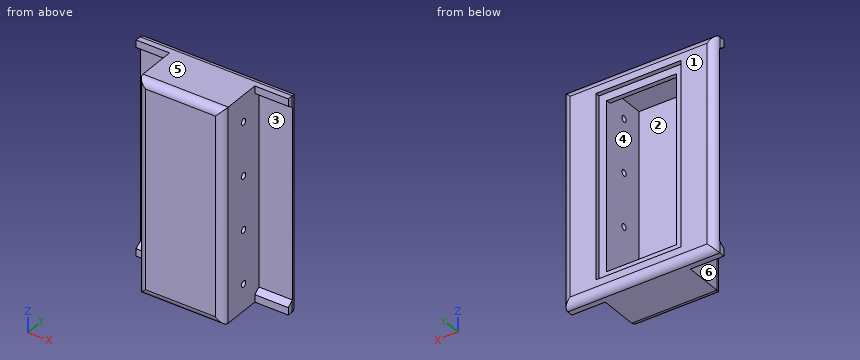
```python
from build123d import *

# Parameters (mm, degrees)
SKETCH1_W           = 200
SKETCH1_H           = 150
BOSS_EXTRUDE1_DEPTH = 280
SKETCH2_W           = 44
SKETCH2_H           = 60
SKETCH2_W_2         = 34
SKETCH2_H_2         = 72.5
CUT_EXTRUDE1_DEPTH  = 280
CUT_EXTRUDE5_DEPTH  = 200
CUT_EXTRUDE8_DEPTH  = 44
CUT_EXTRUDE9_DEPTH  = 44
SKETCH6_W           = 112
SKETCH6_H           = 52.5
CUT_EXTRUDE7_DEPTH  = 280
FILLET1_START       = -100
FILLET1_DEPTH       = 200
FILLET1_START_2     = -76
FILLET1_2_DEPTH     = 10
FILLET1_START_3     = 66
FILLET1_3_DEPTH     = 10
FILLET1_START_4     = -66
FILLET1_4_DEPTH     = 132
FILLET1_START_5     = -281
FILLET1_5_DEPTH     = 282
SKETCH8_W           = 152
SKETCH8_H           = 72.5
CUT_EXTRUDE10_DEPTH = 280
SKETCH9_W           = 111.98598877
SKETCH9_H           = 241.482238642
SKETCH9_W_2         = 91.98598877
SKETCH9_H_2         = 221.482238642
SKETCH9_H_3         = 10
CUT_EXTRUDE11_DEPTH = 6
SKETCH9_3_W         = 45.992994385
SKETCH9_3_H         = 221.482238642
CUT_EXTRUDE12_DEPTH = 67
CUT_EXTRUDE13_START = -12
SKETCH9_7_W         = 91.98598877
SKETCH9_7_H         = 9.258880679
CUT_EXTRUDE13_DEPTH = 55
CUT_EXTRUDE14_START = -12
SKETCH9_9_W         = 91.98598877
SKETCH9_9_H         = 10
CUT_EXTRUDE14_DEPTH = 55
CUT_EXTRUDE15_REACH = 331.182
SKETCH11_R          = 4


with BuildPart() as part:
    # Sketch1 → Boss-Extrude1 (new body)
    with BuildSketch(Plane.XY):
        Rectangle(SKETCH1_W, SKETCH1_H)
    extrude(amount=-BOSS_EXTRUDE1_DEPTH)

    # Sketch2 → Cut-Extrude1 (cut)
    with BuildSketch(Plane.XY):
        with Locations((78, -45)):
            Rectangle(SKETCH2_W, SKETCH2_H)
        with Locations((-78, -45)):
            Rectangle(SKETCH2_W, SKETCH2_H)
        with Locations((83, 38.75)):
            Rectangle(SKETCH2_W_2, SKETCH2_H_2)
        with Locations((-83, 38.75)):
            Rectangle(SKETCH2_W_2, SKETCH2_H_2)
    extrude(amount=-CUT_EXTRUDE1_DEPTH, mode=Mode.SUBTRACT)

    # Sketch3 → Cut-Extrude5 (cut)
    with BuildSketch(Plane.ZY.offset(100)):
        Polygon((-280, 2.5), (-274.399041425, 2.5), (-252, 2.5), (-218.971094498, 75), (-280, 75), align=None)
        Polygon((-236.455453487, 12.5), (-168.766953205, 12.5), (-60.438488841, 12.5), (-94.602997447, 65), (-144.84946991, 65), (-212.537970192, 65), align=None)
        Polygon((-89.179559504, 75), (-42, 2.5), (-5.600958575, 2.5), (0, 2.5), (0, 75), align=None)
    extrude(amount=-CUT_EXTRUDE5_DEPTH, mode=Mode.SUBTRACT)

    # Sketch5 → Cut-Extrude8 (cut)
    with BuildSketch(Plane.ZY.offset(100)):
        Polygon((-264.773291637, -7.125749789), (-270.374250211, -15), (-140, -15), (-140, -7.125749789), align=None)
        Polygon((-15.226708363, -7.125749789), (-140, -7.125749789), (-140, -15), (-9.625749789, -15), align=None)
    extrude(amount=-CUT_EXTRUDE8_DEPTH, mode=Mode.SUBTRACT)

    # Sketch7 → Cut-Extrude9 (cut)
    with BuildSketch(Plane(origin=(100, 0, 0), x_dir=(0, 0, -1), z_dir=(1, 0, 0))):
        Polygon((9.625749789, -15), (15.226708363, -7.125749789), (264.773291637, -7.125749789), (270.374250211, -15), align=None)
    extrude(amount=-CUT_EXTRUDE9_DEPTH, mode=Mode.SUBTRACT)

    # Sketch6 → Cut-Extrude7 (cut)
    with BuildSketch(Plane.XY):
        with Locations((0, 38.75)):
            Rectangle(SKETCH6_W, SKETCH6_H)
    extrude(amount=-CUT_EXTRUDE7_DEPTH, mode=Mode.SUBTRACT)

    # Fillet1: read off the stored shape, not the designer's step
    # Fillet1 outline → Fillet1 (cut)
    with BuildSketch(Plane.YZ.offset(FILLET1_START)):
        with BuildLine():
            Line((-75, 0), (-75, -10))
            ThreePointArc((-75, -10), (-72.071067812, -2.928932188), (-65, 0))
            Line((-65, 0), (-75, 0))
        make_face()
        with BuildLine():
            ThreePointArc((-65, -280), (-72.071067812, -277.071067812), (-75, -270))
            Line((-75, -270), (-75, -280))
            Line((-75, -280), (-65, -280))
        make_face()
        with BuildLine():
            Line((2.5, 0), (-7.5, 0))
            ThreePointArc((-7.5, 0), (-0.428932188, -2.928932188), (2.5, -10))
            Line((2.5, -10), (2.5, 0))
        make_face()
        with BuildLine():
            ThreePointArc((2.5, -270), (-0.428932188, -277.071067812), (-7.5, -280))
            Line((-7.5, -280), (2.5, -280))
            Line((2.5, -280), (2.5, -270))
        make_face()
        with BuildLine():
            Line((75, -89.179559504), (70.454316835, -86.221444616))
            ThreePointArc((70.454316835, -86.221444616), (73.790425711, -89.835564613), (75, -94.602997447))
            Line((75, -94.602997447), (75, -89.179559504))
        make_face()
        with BuildLine():
            ThreePointArc((75, -212.537970192), (73.410042611, -217.948255145), (69.145763344, -221.638115591))
            Line((69.145763344, -221.638115591), (75, -218.971094498))
            Line((75, -218.971094498), (75, -212.537970192))
        make_face()
    extrude(amount=FILLET1_DEPTH, mode=Mode.SUBTRACT)

    # Fillet1 2 outline → Fillet1 2 (add)
    with BuildSketch(Plane.YZ.offset(FILLET1_START_2)):
        with BuildLine():
            ThreePointArc((7.045683165, -44.958114888), (3.709574289, -41.343994891), (2.5, -36.576562057))
            Line((2.5, -36.576562057), (2.5, -258.433124306))
            ThreePointArc((2.5, -258.433124306), (4.089957389, -253.022839352), (8.354236656, -249.332978906))
            Line((8.354236656, -249.332978906), (69.145763344, -221.638115591))
            ThreePointArc((69.145763344, -221.638115591), (73.410042611, -217.948255145), (75, -212.537970192))
            Line((75, -212.537970192), (75, -94.602997447))
            ThreePointArc((75, -94.602997447), (73.790425711, -89.835564613), (70.454316835, -86.221444616))
            Line((70.454316835, -86.221444616), (7.045683165, -44.958114888))
        make_face()
    extrude(amount=FILLET1_2_DEPTH)

    # Fillet1 3 outline → Fillet1 3 (add)
    with BuildSketch(Plane.YZ.offset(FILLET1_START_3)):
        with BuildLine():
            ThreePointArc((7.045683165, -44.958114888), (3.709574289, -41.343994891), (2.5, -36.576562057))
            Line((2.5, -36.576562057), (2.5, -258.433124306))
            ThreePointArc((2.5, -258.433124306), (4.089957389, -253.022839352), (8.354236656, -249.332978906))
            Line((8.354236656, -249.332978906), (69.145763344, -221.638115591))
            ThreePointArc((69.145763344, -221.638115591), (73.410042611, -217.948255145), (75, -212.537970192))
            Line((75, -212.537970192), (75, -94.602997447))
            ThreePointArc((75, -94.602997447), (73.790425711, -89.835564613), (70.454316835, -86.221444616))
            Line((70.454316835, -86.221444616), (7.045683165, -44.958114888))
        make_face()
    extrude(amount=FILLET1_3_DEPTH)

    # Fillet1 4 outline → Fillet1 4 (add)
    with BuildSketch(Plane.YZ.offset(FILLET1_START_4)):
        with BuildLine():
            ThreePointArc((7.045683165, -44.958114888), (3.709574289, -41.343994891), (2.5, -36.576562057))
            Line((2.5, -36.576562057), (2.5, -42))
            Line((2.5, -42), (7.045683165, -44.958114888))
        make_face()
        with BuildLine():
            Line((2.5, -252), (2.5, -258.433124306))
            ThreePointArc((2.5, -258.433124306), (4.089957389, -253.022839352), (8.354236656, -249.332978906))
            Line((8.354236656, -249.332978906), (2.5, -252))
        make_face()
    extrude(amount=FILLET1_4_DEPTH)

    # Fillet1 5 outline → Fillet1 5 (cut)
    with BuildSketch(Plane.XY.offset(FILLET1_START_5)):
        with BuildLine():
            ThreePointArc((56, 75), (63.071067812, 72.071067812), (66, 65))
            Line((66, 65), (66, 12.5))
            ThreePointArc((66, 12.5), (68.928932188, 5.428932188), (76, 2.5))
            Line((76, 2.5), (76, 75))
            Line((76, 75), (56, 75))
        make_face()
        with BuildLine():
            ThreePointArc((-66, 65), (-63.071067812, 72.071067812), (-56, 75))
            Line((-56, 75), (-76, 75))
            Line((-76, 75), (-76, 2.5))
            ThreePointArc((-76, 2.5), (-68.928932188, 5.428932188), (-66, 12.5))
            Line((-66, 12.5), (-66, 65))
        make_face()
        with BuildLine():
            Line((100, 2.5), (90, 2.5))
            ThreePointArc((90, 2.5), (97.071067812, -0.428932188), (100, -7.5))
            Line((100, -7.5), (100, 2.5))
        make_face()
        with BuildLine():
            Line((-90, 2.5), (-100, 2.5))
            Line((-100, 2.5), (-100, -7.5))
            ThreePointArc((-100, -7.5), (-97.071067812, -0.428932188), (-90, 2.5))
        make_face()
        with BuildLine():
            Line((56, -75), (56, -65))
            ThreePointArc((56, -65), (53.071067812, -72.071067812), (46, -75))
            Line((46, -75), (56, -75))
        make_face()
        with BuildLine():
            ThreePointArc((-46, -75), (-53.071067812, -72.071067812), (-56, -65))
            Line((-56, -65), (-56, -75))
            Line((-56, -75), (-46, -75))
        make_face()
    extrude(amount=FILLET1_5_DEPTH, mode=Mode.SUBTRACT)

    # Sketch8 → Cut-Extrude10 (cut)
    with BuildSketch(Plane.XY):
        with Locations((0, 38.75)):
            Rectangle(SKETCH8_W, SKETCH8_H)
    extrude(amount=-CUT_EXTRUDE10_DEPTH, mode=Mode.SUBTRACT)

    # Sketch9 → Cut-Extrude11 (cut)
    # profile 1 of 4: a face of its own
    with BuildSketch(Plane(origin=(0, 2.5, 0), x_dir=(1, 0, 0), z_dir=(0, 1, 0))):
        with Locations((0, 140)):
            Rectangle(SKETCH9_W, SKETCH9_H)
        with Locations((0, 140)):
            Rectangle(SKETCH9_W_2, SKETCH9_H_2, mode=Mode.SUBTRACT)
    # profile 2 of 4: a face of its own
    with BuildSketch(Plane(origin=(0, 2.5, 0), x_dir=(1, 0, 0), z_dir=(0, 1, 0))):
        Polygon((55.992994385, 260.741119321), (45.992994385, 260.741119321), (45.992994385, 250.741119321), (45.992994385, 29.258880679), (45.992994385, 19.258880679), (55.992994385, 19.258880679), align=None)
    # profile 3 of 4: a face of its own
    with BuildSketch(Plane(origin=(0, 2.5, 0), x_dir=(1, 0, 0), z_dir=(0, 1, 0))):
        with Locations((0, 255.741119321)):
            Rectangle(SKETCH9_W_2, SKETCH9_H_3)
    # profile 4 of 4: a face of its own
    with BuildSketch(Plane(origin=(0, 2.5, 0), x_dir=(1, 0, 0), z_dir=(0, 1, 0))):
        with Locations((0, 24.258880679)):
            Rectangle(SKETCH9_W_2, SKETCH9_H_3)
    extrude(amount=-CUT_EXTRUDE11_DEPTH, mode=Mode.SUBTRACT)

    # Sketch9<3> → Cut-Extrude12 (cut)
    with BuildSketch(Plane(origin=(0, 2.5, 0), x_dir=(1, 0, 0), z_dir=(0, 1, 0))):
        with Locations((-22.996497193, 140)):
            Rectangle(SKETCH9_3_W, SKETCH9_3_H)
        with Locations((22.996497193, 140)):
            Rectangle(SKETCH9_3_W, SKETCH9_3_H)
    extrude(amount=-CUT_EXTRUDE12_DEPTH, mode=Mode.SUBTRACT)

    # Sketch9<7> → Cut-Extrude13 (cut)
    with BuildSketch(Plane(origin=(0, 2.5, 0), x_dir=(1, 0, 0), z_dir=(0, 1, 0)).offset(CUT_EXTRUDE13_START)):
        with Locations((0, 265.370559661)):
            Rectangle(SKETCH9_7_W, SKETCH9_7_H)
        with Locations((0, 14.62944034)):
            Rectangle(SKETCH9_7_W, SKETCH9_7_H)
    extrude(amount=-CUT_EXTRUDE13_DEPTH, mode=Mode.SUBTRACT)

    # Sketch9<9> → Cut-Extrude14 (cut)
    with BuildSketch(Plane(origin=(0, 2.5, 0), x_dir=(1, 0, 0), z_dir=(0, 1, 0)).offset(CUT_EXTRUDE14_START)):
        with Locations((0, 255.741119321)):
            Rectangle(SKETCH9_9_W, SKETCH9_9_H)
        with Locations((0, 24.258880679)):
            Rectangle(SKETCH9_9_W, SKETCH9_9_H)
    extrude(amount=-CUT_EXTRUDE14_DEPTH, mode=Mode.SUBTRACT)

    # Cut-Extrude15: up to this face of the body (flat: up to its plane)
    cut_extrude15_end = Plane(part.part.faces().sort_by_distance((56, -36.372089238, -140))[0])
    # Sketch11 → Cut-Extrude15 (cut, up to the picked face)
    with BuildSketch(Plane.ZY.offset(56), mode=Mode.PRIVATE) as cut_extrude15_sk1:
        with Locations((-35, -36.062874894)):
            Circle(SKETCH11_R)
    cut_extrude15_tool1 = split(extrude(cut_extrude15_sk1.sketch, amount=-CUT_EXTRUDE15_REACH, mode=Mode.PRIVATE), bisect_by=cut_extrude15_end, keep=Keep.BOTH, mode=Mode.PRIVATE)
    # Sketch11 → Cut-Extrude15 (cut, up to the picked face)
    with BuildSketch(Plane.ZY.offset(56), mode=Mode.PRIVATE) as cut_extrude15_sk2:
        with Locations((-105, -36.062874894)):
            Circle(SKETCH11_R)
    cut_extrude15_tool2 = split(extrude(cut_extrude15_sk2.sketch, amount=-CUT_EXTRUDE15_REACH, mode=Mode.PRIVATE), bisect_by=cut_extrude15_end, keep=Keep.BOTH, mode=Mode.PRIVATE)
    # Sketch11 → Cut-Extrude15 (cut, up to the picked face)
    with BuildSketch(Plane.ZY.offset(56), mode=Mode.PRIVATE) as cut_extrude15_sk3:
        with Locations((-175, -36.062874894)):
            Circle(SKETCH11_R)
    cut_extrude15_tool3 = split(extrude(cut_extrude15_sk3.sketch, amount=-CUT_EXTRUDE15_REACH, mode=Mode.PRIVATE), bisect_by=cut_extrude15_end, keep=Keep.BOTH, mode=Mode.PRIVATE)
    # Sketch11 → Cut-Extrude15 (cut, up to the picked face)
    with BuildSketch(Plane.ZY.offset(56), mode=Mode.PRIVATE) as cut_extrude15_sk4:
        with Locations((-245, -36.062874894)):
            Circle(SKETCH11_R)
    cut_extrude15_tool4 = split(extrude(cut_extrude15_sk4.sketch, amount=-CUT_EXTRUDE15_REACH, mode=Mode.PRIVATE), bisect_by=cut_extrude15_end, keep=Keep.BOTH, mode=Mode.PRIVATE)
    add(cut_extrude15_tool1.solids().sort_by(Axis((-56, -36.062875, -35), (1, 0, 0)))[0], mode=Mode.SUBTRACT)
    add(cut_extrude15_tool2.solids().sort_by(Axis((-56, -36.062875, -105), (1, 0, 0)))[0], mode=Mode.SUBTRACT)
    add(cut_extrude15_tool3.solids().sort_by(Axis((-56, -36.062875, -175), (1, 0, 0)))[0], mode=Mode.SUBTRACT)
    add(cut_extrude15_tool4.solids().sort_by(Axis((-56, -36.062875, -245), (1, 0, 0)))[0], mode=Mode.SUBTRACT)


solid = part.part
```
Model file for the job. Use its own axes, mm. Face numbers are marked on the shaded views. A direction names the side the tool comes from. Give positions to 0.01 mm unless a question says otherwise; leave off trailing zeros. Write each loop counter-clockwise with the first axis right and the second up, starting at its lowest first coordinate (ties: lowest second). Pieces come first, ordered by that corner, then holes. Notation, with made-up numbers: (-26, 59.5) - (18, 59.5) arc R27 cw to (18, 92.5) - close; hole circle Ø1 at (34, -31.75). An arc over 180 degrees is marked (long way). One line per question, with ' | ' between items. Start each with the question number.
(1) Slice it at D-D on z = -152. Write the cut outline in (x, y).
(2) Slice it at B-B on y = -28.5. Write the cut outline in (x, z), plus the area to 3 significant figures.
(3) Two-plate mould, pull along X, no slides. Class the marked faces 4, 5 and 6: +X half, -X half, draft (parallel to the pull), parting line (faces both ways), or undercut.
(4) Slice it at A-A on z = -245. Write the cut outline in (x, y).
(5) Slice it at C-C on x = -69. Write the cut outline in (y, z).
(6) Pin check, flat tips, straight feed: P1, Ø1.5, axis at x = -19.5, y = -5.5, coming from the -Z side; P2, Ø1.5, axis at y = -39.5, z = -218, coming from the +X side; P3, Ø3, axis at x = 22, y = -0.5, coming from the +Z side. Stop position of each tip, or through.
(7) Wall check: line 1 along X through (y, z) = (-23, -123); line 2 along Z through (x, y) = (-33, -38); line 3 along X through (y, z) = (-7, -142). Give the ranges that are in metal, low to high. Write a range as from..to.
(8) 3-axis set-ups, long thin cutter, end or side, ignore diameter. For the marked faces 1, 2 and 3: which of +Z, -Z, +X, -X, +Y, -Y reach the whole face in a straight line?
Results below:
1) outline: (-99.99, -7.13) - (-56, -7.13) - (-56, -65) arc R10 ccw to (-46, -75) - (46, -75) arc R10 ccw to (56, -65) - (56, -7.13) - (99.99, -7.13) arc R10 ccw to (90, 2.5) - (55.99, 2.5) - (55.99, -3.5) - (45.99, -3.5) - (45.99, -64.5) - (-45.99, -64.5) - (-45.99, -3.5) - (-55.99, -3.5) - (-55.99, 2.5) - (-90, 2.5) arc R10 ccw to start
2) outline: (-56, -280) - (56, -280) - (56, 0) - (-56, 0) - close; hole (-45.99, -270) - (45.99, -270) - (45.99, -10) - (-45.99, -10) - close | area: 7,440 mm^2
3) face 4: undercut | face 5: draft | face 6: -X half
4) outline: (-99.99, -7.13) - (-56, -7.13) - (-56, -32.06) - (-45.99, -32.06) - (-45.99, -3.5) - (-55.99, -3.5) - (-55.99, 2.5) - (-90, 2.5) arc R10 ccw to start; (-56, -65) arc R10 ccw to (-46, -75) - (46, -75) arc R10 ccw to (56, -65) - (56, -40.06) - (45.99, -40.06) - (45.99, -64.5) - (-45.99, -64.5) - (-45.99, -40.06) - (-56, -40.06) - close; (45.99, -32.06) - (56, -32.06) - (56, -7.13) - (99.99, -7.13) arc R10 ccw to (90, 2.5) - (55.99, 2.5) - (55.99, -3.5) - (45.99, -3.5) - close
5) outline: (-15, -280) - (-7.5, -280) arc R10 ccw to (2.5, -270) - (2.5, -10) arc R10 ccw to (-7.5, 0) - (-15, 0) - (-15, -9.63) - (-7.13, -15.23) - (-7.13, -264.77) - (-15, -270.37) - close
6) P1: z = -279.92 | P2: x = 56 | P3: z = -1.65
7) line 1: -56..-45.99, 45.99..56 | line 2: -280..-270, -10..0 | line 3: -99.99..-45.99, 45.99..99.99
8) face 1: +Z, -Z, +X, -X, +Y | face 2: none | face 3: +X, -Y
